from build123d import *


with BuildPart() as f3:
    # F0 (on Front) → F3 section 0
    with BuildSketch(Plane.XZ, mode=Mode.PRIVATE) as f3_s0:
        Polygon((22.694931, 59.195888), (-32.13115, 54.651644), (-62.76182, 8.953598), (-46.13156, -43.48669), (5.236706, -63.180614), (52.661626, -35.298246), (60.431267, 19.16442), align=None)
    loft([f3_s0.sketch, Vertex(0, 100, -4.40801)])


solid = f3.part
Work out the finished part from the listing and answer in its coordinate system (mm). Coordinates: 2 decimals unless noted, no trailing zeros. Loops run counter-clockwise (first coordinate to the right, second up) from the corner with the lowest first, then second, coordinate; pieces in that order, holes last. Notation, with made-up numbers: M -15.75,-12.75 L 26.25,-12.75 A11 cw 26.25,-7.75 Z; hole C 75,-3.5 d4. An arc over 180 degrees is marked long. Answer in a Markdown table with one row per item. Add a question column.
1. Find section B-B, the plane x = 12. Write down the section's boundary in (y, z), then the cut area to 3 significant figures.
2. Find section A-A, the plane y = 63.5. Write down the section's boundary in (x, z).
3. Find section D-D, the plane y = 16.5. Write down the section's boundary in (x, z), then the cut area to 3 significant figures.
4. Consider L1, parallel to Z at x = -1, y = 11; L2, parallel to Y at x = -37, z = -33; L3, parallel to X at y = 20, z = -28. Determine where each line is inside the solid, lowest interval first.
5. Flat-ended cylindrical pins translate along their axes: P1, Ø12, axis at x = 26, y = 38.5, coming from the +Z side; P2, Ø2, axis at y = 47, z = 1.5, coming from the +X side; P3, Ø10, axis at x = 18.5, y = 47, coming from the +Z side. Find the tip coordinate at first contact, or state that the pin passes through.
6. Find section C-C, the plane z = 17. Write down the section's boundary in (x, y), then the cut area to 3 significant figures.
Reported:
| question | item | result |
|---|---|---|
| 1 | outline | M 0,-59.2 L 77.21,-11.45 L 80.14,0.27 L 47.12,29.22 L 0,58.31 Z |
| 1 | area | 5,290 mm^2 |
| 2 | outline | M -22.91,0.47 L -16.84,-18.67 L 1.91,-25.86 L 19.22,-15.68 L 22.06,4.2 L 8.28,18.81 L -11.73,17.15 Z |
| 3 | outline | M -52.41,6.75 L -38.52,-37.04 L 4.37,-53.48 L 43.97,-30.2 L 50.46,15.27 L 18.95,48.7 L -26.83,44.91 Z |
| 3 | area | 7,670 mm^2 |
| 4 | L1 | z = -54.55 to 50.44 |
| 4 | L2 | y = 0 to 21.29 |
| 4 | L3 | x = -39.34 to 42.29 |
| 5 | P1 | stops at z = 30.19 |
| 5 | P2 | stops at x = 31.68 |
| 5 | P3 | stops at z = 29.32 |
| 6 | outline | M -57.37,0 L 60.12,0 L 54.88,9.18 L 7.64,66.34 L -11.65,63.75 Z |
| 6 | area | 4,520 mm^2 |
